Here's how the part is built. I have some questions about the finished solid (model axes, mm). Face numbers are marked on the shaded views. Round coordinates to 2 decimals unless told otherwise and drop trailing zeros. Loops run counter-clockwise (first coordinate to the right, second up) from the corner with the lowest first, then second, coordinate; pieces in that order, holes last. Notation, with made-up numbers: (43, 53) - (98, 53) arc R8 ccw to (98, 62) - close; hole circle Ø4 at (-21.5, -36.5). An arc over 180 degrees is marked (long way). Return JSON: item names as keys, results as strings. Group by question number.
Autodesk Inventor part; units mm, degrees
ref_plane "YZ Plane" through (0, 0, 0) normal (1, 0, 0) x (0, 1, 0)
ref_plane "XZ Plane" through (0, 0, 0) normal (0, 1, 0) x (-1, 0, 0)
ref_plane "XY Plane" through (0, 0, 0) normal (0, 0, 1) x (1, 0, 0)
sketch "Sketch1" plane through (0, 0, 0) normal (0, 1, 0) x (-1, 0, 0)
  circle A0 centre (0, 0) radius 41.275
  dimension "d0" = 82.55
extrude "Extrusion1" add sketch "Sketch1" along normal blind 0.75
sketch "Sketch2" plane through (0, 0.75, 0) normal (0, 1, 0) x (1, 0, 0)
  circle A0 centre (0, 0) radius 31.75
  circle A1 centre (0, 0) radius 41.275
  circle A2 centre (0, 0) radius 32.75
  circle A3 centre (0, 0) radius 40.275
  dimension "d3" = 63.5
  dimension "d4" = 1
  dimension "d5" = 1
extrude "Extrusion2" add sketch "Sketch2" along normal blind 25.4
fillet "Fillet1" radius 0.5 1 edges at (-32.75, 26.15, 0)
sketch "Sketch3" plane through (0, 0.75, 0) normal (0, 1, 0) x (1, 0, 0)
  circle A0 centre (0, 0) radius 17.4625 construction
  line L0 (0, 0) -> (0, -17.4625) construction
  circle A1 centre (0, -17.4625) radius 1.905
  circle A2 centre (15.123, -8.7313) radius 1.905
  circle A3 centre (15.123, 8.7312) radius 1.905
  circle A4 centre (0, 17.4625) radius 1.905
  circle A5 centre (-15.123, 8.7313) radius 1.905
  circle A6 centre (-15.123, -8.7312) radius 1.905
  dimension "d9" = 34.925
  dimension "d10" = 3.81
  dimension "d13" = 360
extrude "Extrusion3" cut sketch "Sketch3" against normal through all
sketch "Sketch4" plane through (0, 0.75, 0) normal (0, 1, 0) x (1, 0, 0)
  circle A0 centre (0, 0) radius 3.4925
  dimension "d17" = 6.985
extrude "Extrusion4" add sketch "Sketch4" along normal blind 9.525
properties part number "Mold - Wheel"
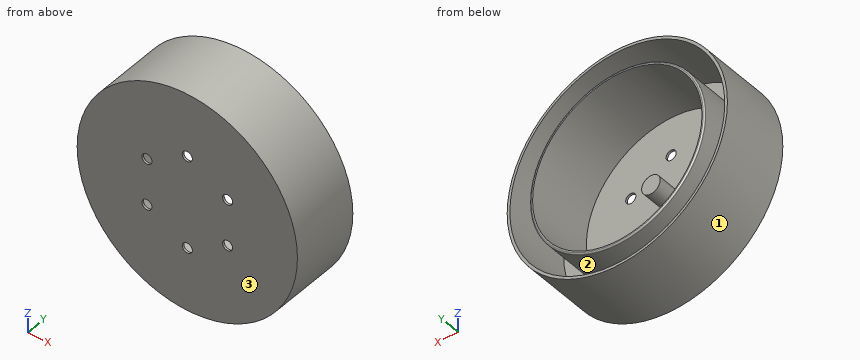
Q1. Imagine slicing it at C-C, the plane y = 14.5. List the corners of the cut face in (x, z) for me (3 decimals).
Q2. Imagine slicing it at B-B, the plane y = 8.75. Give the number of separate pieces and of enclosed holes in the cut face, and give its area (3 significant figures).
Q3. Will these pins go through, and if not, where does the flat tip stop? pin 1 Ø3 at (x, z) = (0, 17.46) entering from -Y; pin 2 Ø3 at (x, z) = (-24, -7) entering from +Y; pin 3 Ø2 at (x, z) = (1.5, -0.5) entering from +Y (3 decimals); pin 4 Ø1 at (y, z) = (12.5, 29) entering from -X.
Q4. Please list where these lines run through material, in increasing order: line 1 (Z direction, x = -6.5, y = 2); line 2 (X direction, y = 18, z = -29.5); line 3 (X direction, y = 21.25, z = -3).
Q5. If we mould it in two halves opening along X, with no side actions, what happens to the marked faces 1, 2 and 3? For each: +X half, -X half, draft (parallel to the pull), parting line (faces both ways), or undercut.
Output values:
{
 "1": {"outline": "circle Ø82.55 at (0, 0); circle Ø65.5 at (0, 0); hole circle Ø80.55 at (0, 0); hole circle Ø63.5 at (0, 0)"},
 "2": {"separate pieces": "3", "enclosed holes": "2", "area": "497 mm^2"},
 "3": {"pin 1": "passes through", "pin 2": "stops at y = 0.75", "pin 3": "stops at y = 10.275", "pin 4": "stops at x = -29.86"},
 "4": {"line 1": "z = -40.76 to -39.75, -32.1 to -31.08, 31.08 to 32.1, 39.75 to 40.76", "line 2": "x = -28.87 to -27.42, -14.22 to -11.74, 11.74 to 14.22, 27.42 to 28.87", "line 3": "x = -41.17 to -40.16, -32.61 to -31.61, 31.61 to 32.61, 40.16 to 41.17"},
 "5": {"face 1": "parting line", "face 2": "undercut", "face 3": "draft"}
}
